Source: three-view drawing plus pictorial views. Frame: mm from the lowest corner of the part. A direction names the side the tool comes from. Give positions to 0.01 mm unless a question says otherwise; leave off trailing zeros. Order: outer loops, then holes, each group sorted by start corner. A loop starts at its lowest first (then second) coordinate and runs counter-clockwise, first axis right, second up. Notation, with made-up numbers: M 13.5,-21 L 28.5,-21 A29 cw 28.5,15 Z; hole C 46.25,-20 d6. An arc over 180 degrees is marked long. Use CSV: the item, a comma, the result in double quotes.
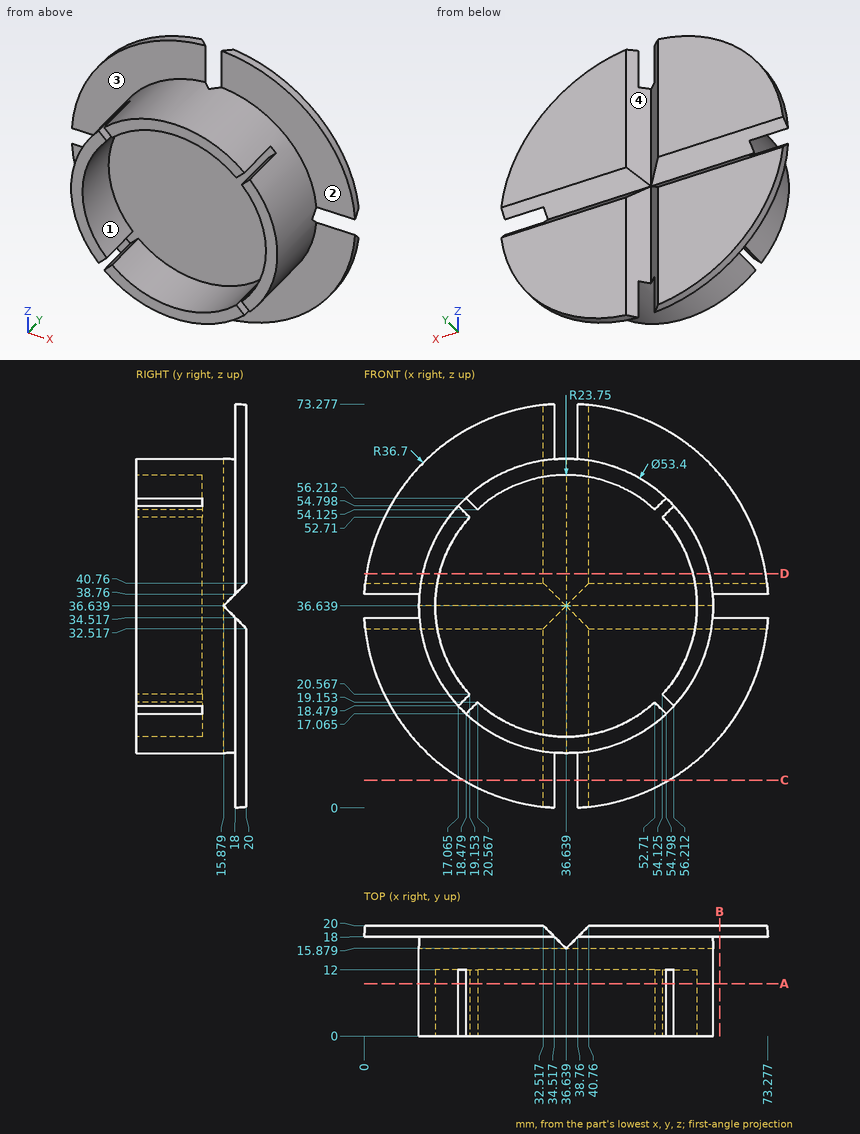
1. Pin query (flat end, axial travel): pin 1 Ø8 at (x, y) = (47.5, 17.5) entering from +Z (1 decimal); pin 2 Ø2 at (x, z) = (57.5, 39.5) entering from -Y; pin 3 Ø2 at (x, y) = (20, 13) entering from +Z. Return the tip coordinate at first contact, or that it passes through.
Answer:
pin 1,"z = 72.7"
pin 2,"y = 12"
pin 3,"z = 58.28"
2. Section A-A, the plane y = 9.5. Give the number of separate pieces and of enclosed holes in the cut face, plus the area to 3 significant figures.
Answer:
separate pieces,"4"
enclosed holes,"0"
area,"444 mm2"
3. Section D-D, the plane z = 42.5. Return the cut outline in (x, y).
Answer:
outline,"M 0.41,18 L 10.59,18 L 10.59,0 L 13.62,0 L 13.62,12 L 59.65,12 L 59.65,0 L 62.69,0 L 62.69,18 L 72.87,18 L 72.87,20 L 40.76,20 L 36.64,15.88 L 32.52,20 L 0.41,20 Z"
4. Section C-C, the plane z = 5. Return the cut outline in (x, y).
Answer:
outline,"M 18.04,18 L 34.52,18 L 32.52,20 L 18.04,20 Z; M 38.76,18 L 55.24,18 L 55.24,20 L 40.76,20 Z"
5. Reachability of the marked faces 1, 2, 3 and 4 from +Z, -Z, +X, -X, +Y, -Y: full face, straight path, thin tool, end or side. Return the list, or none.
Answer:
face 1,"-Y"
face 2,"+Z, +X, -Y"
face 3,"+Z, -X, -Y"
face 4,"+Z, -Z, +Y"
6. Section B-B, the plane x = 64.5. Return the cut outline in (y, z).
Answer:
outline,"M 18,12.75 L 20,12.75 L 20,32.52 L 18,34.52 Z; M 18,38.76 L 20,40.76 L 20,60.53 L 18,60.53 Z"
7. Line query: line 1 (Y direction, x = 29, z = 4); line 2 (X direction, y = 6, z = 44) (1 decimal); line 3 (X direction, y = 5.75, z = 18) (1 decimal). Output: solid intervals per line, ascending.
Answer:
line 1,"18 to 20"
line 2,"11 to 14.1, 59.2 to 62.3"
line 3,"19.4 to 21.9, 51.4 to 53.9"
